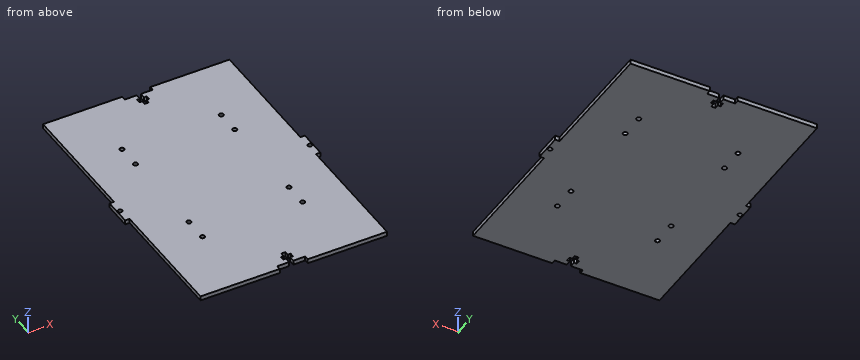
```python
from build123d import *

# Parameters (mm, degrees)
SKETCH1_W           = 139.7
SKETCH1_H           = 200.02
BOSS_EXTRUDE1_DEPTH = 3.18
SKETCH2_R           = 1.5
SKETCH2_W           = 3.18
SKETCH2_H           = 90.135
CUT_EXTRUDE1_DEPTH  = 4.18
SKETCH3_R           = 1.59
CUT_EXTRUDE2_DEPTH  = 4.18
SKETCH4_R           = 1.59
CUT_EXTRUDE3_DEPTH  = 4.18


with BuildPart() as part:
    # Sketch1 → Boss-Extrude1 (new body)
    with BuildSketch(Plane.XY):
        Rectangle(SKETCH1_W, SKETCH1_H)
    extrude(amount=BOSS_EXTRUDE1_DEPTH)

    # Sketch2 → Cut-Extrude1 (cut, through all)
    with BuildSketch(Plane.XY.offset(3.18)):
        with Locations((-67.85, 0)):
            Circle(SKETCH2_R)
        with Locations((67.85, 0)):
            Circle(SKETCH2_R)
        Polygon((-10, 100.01), (10, 100.01), (10, 96.83), (1.5, 96.83), (1.5, 92.83), (3.5, 92.83), (3.5, 89.83), (1.5, 89.83), (1.5, 86.83), (-1.5, 86.83), (-1.5, 89.83), (-3.5, 89.83), (-3.5, 92.83), (-1.5, 92.83), (-1.5, 96.83), (-10, 96.83), align=None)
        Polygon((-10, -100.01), (-10, -96.83), (-1.5, -96.83), (-1.5, -92.83), (-3.5, -92.83), (-3.5, -89.83), (-1.5, -89.83), (-1.5, -86.83), (1.5, -86.83), (1.5, -89.83), (3.5, -89.83), (3.5, -92.83), (1.5, -92.83), (1.5, -96.83), (10, -96.83), (10, -100.01), align=None)
        with Locations((-68.26, 54.9425)):
            Rectangle(SKETCH2_W, SKETCH2_H)
        with Locations((-68.26, -54.9425)):
            Rectangle(SKETCH2_W, SKETCH2_H)
        with Locations((68.26, -54.9425)):
            Rectangle(SKETCH2_W, SKETCH2_H)
        with Locations((68.26, 54.9425)):
            Rectangle(SKETCH2_W, SKETCH2_H)
    extrude(amount=-CUT_EXTRUDE1_DEPTH, mode=Mode.SUBTRACT)

    # Sketch3 → Cut-Extrude2 (cut, through all)
    with BuildSketch(Plane(origin=(0, 0, 0), x_dir=(-1, 0, 0), z_dir=(0, 0, -1))):
        with Locations((-35.67127699, -47.963396943)):
            Circle(SKETCH3_R)
        with Locations((-35.67127699, -30.777287406)):
            Circle(SKETCH3_R)
    extrude(amount=-CUT_EXTRUDE2_DEPTH, mode=Mode.SUBTRACT)

    # Sketch4 → Cut-Extrude3 (cut, through all)
    with BuildSketch(Plane(origin=(0, 0, 0), x_dir=(-1, 0, 0), z_dir=(0, 0, -1))):
        with Locations((-34.750723073, 53.780323187)):
            Circle(SKETCH4_R)
        with Locations((-34.750723073, 36.59421365)):
            Circle(SKETCH4_R)
        with Locations((36.249784221, 53.780323187)):
            Circle(SKETCH4_R)
        with Locations((36.249784221, 36.59421365)):
            Circle(SKETCH4_R)
        with Locations((35.983928162, -30.777287406)):
            Circle(SKETCH4_R)
        with Locations((35.983928162, -47.963396943)):
            Circle(SKETCH4_R)
        with Locations((-35.67127699, -30.777287406)):
            Circle(SKETCH4_R)
        with Locations((-35.67127699, -47.963396943)):
            Circle(SKETCH4_R)
    extrude(amount=-CUT_EXTRUDE3_DEPTH, mode=Mode.SUBTRACT)


solid = part.part
```
Geometry check sheet. Reference: the model listing, model coordinates, mm. Round coordinates to 2 decimals unless told otherwise and drop trailing zeros. Order: outer loops, then holes, each group sorted by start corner. A loop starts at its lowest first (then second) coordinate and runs counter-clockwise, first axis right, second up. Notation, with made-up numbers: (53.5, 43) - (66.5, 43) arc R29 cw to (66.5, 67) - close; hole circle Ø4 at (41.5, -22). An arc over 180 degrees is marked (long way). Use a Markdown table: item, result. Add a question column.
1) Thickness scan on line 1 along Y through (x, z) = (-37, 1.7); line 2 along X through (y, z) = (46.5, 0.75); line 3 along X through (y, z) = (-48.5, 2.85). Record the ranges inside material, lowest first.
2) Section check B-B (z = 2.4). Count the separate pieces of the cut face and the enclosed holes in it, then the cut area to 3 significant figures.
3) Section check A-A (y = 19.5). Record the cut outline in (x, z).
4) Gauge pin test, flat ends, axial feed: P1, Ø1.6, axis at x = -2.5, z = 1.5, coming from the +Y side; P2, Ø2, axis at x = -47.5, y = 6, coming from the -Z side; P3, Ø1, axis at y = -94, z = 2, coming from the -X side; P4, Ø1, axis at x = 69, z = 2, coming from the +Y side (3 decimals). Record the tip position at first contact, or that the pin passes through.
5) Section check C-C (x = 8). Record the cut outline in (y, z), then the cut area to 3 significant figures.
Established:
| question | item | result |
|---|---|---|
| 1 | line 1 | -100.01 to -49.19, -46.74 to -32, -29.55 to 35.19, 38 to 52.38, 55.18 to 100.01 |
| 1 | line 2 | -66.67 to 66.67 |
| 1 | line 3 | -66.67 to -37.48, -34.49 to 34.17, 37.17 to 66.67 |
| 2 | separate pieces | 1 |
| 2 | enclosed holes | 10 |
| 2 | area | 26,500 mm2 |
| 3 | outline | (-66.67, 0) - (66.67, 0) - (66.67, 3.18) - (-66.67, 3.18) - close |
| 4 | P1 | y = 96.83 |
| 4 | P2 | z = 0 |
| 4 | P3 | x = -66.67 |
| 4 | P4 | y = 9.875 |
| 5 | outline | (-96.83, 0) - (96.83, 0) - (96.83, 3.18) - (-96.83, 3.18) - close |
| 5 | area | 616 mm2 |
